```python
from build123d import *

# Parameters (mm, degrees)
SKETCH1_R           = 1
BOSS_EXTRUDE1_DEPTH = 9
SKETCH2_R           = 2
SKETCH2_R_2         = 1
BOSS_EXTRUDE3_DEPTH = 4
SKETCH3_R           = 2
BOSS_EXTRUDE4_DEPTH = 12.3
SKETCH4_W           = 8
SKETCH4_H           = 2.3
CUT_EXTRUDE1_DEPTH  = 100


with BuildPart() as part:
    # Sketch1 → Boss-Extrude1 (new body)
    with BuildSketch(Plane.XY):
        with BuildLine():
            Line((37.44618629, 199.100176708), (21.157913115, 198.645068222))
            ThreePointArc((21.157913115, 198.645068222), (19.402812913, 197.854741355), (18.729526359, 196.051500247))
            Line((18.729526359, 196.051500247), (19.122128495, 185.677380061))
            ThreePointArc((19.122128495, 185.677380061), (19.911642331, 183.946998209), (21.690165088, 183.272898624))
            Line((21.690165088, 183.272898624), (46.213174666, 183.958092791))
            ThreePointArc((46.213174666, 183.958092791), (47.16140114, 184.173792868), (47.955590742, 184.734972736))
            Line((47.955590742, 184.734972736), (53.340647935, 190.401756173))
            Line((53.340647935, 190.401756173), (50.421306908, 190.401756173))
            ThreePointArc((50.421306908, 190.401756173), (49.61024665, 190.536976848), (48.886924084, 190.928011166))
            Line((48.886924084, 190.928011166), (39.050394032, 198.574897009))
            ThreePointArc((39.050394032, 198.574897009), (38.293965035, 198.977028229), (37.44618629, 199.100176708))
        make_face()
        with Locations((20.799047924, 194.252293006)):
            Circle(SKETCH1_R, mode=Mode.SUBTRACT)
        with Locations((38.792906294, 194.755057023)):
            Circle(SKETCH1_R, mode=Mode.SUBTRACT)
        with Locations((39.095459561, 186.760388464)):
            Circle(SKETCH1_R, mode=Mode.SUBTRACT)
        with Locations((21.101601191, 186.257624448)):
            Circle(SKETCH1_R, mode=Mode.SUBTRACT)
    extrude(amount=BOSS_EXTRUDE1_DEPTH)

    # Sketch2 → Boss-Extrude3 (add)
    with BuildSketch(Plane.XY.offset(9)):
        with BuildLine():
            Line((61.820501213, 210.938669532), (45.388864845, 193.647390819))
            Line((45.388864845, 193.647390819), (48.886924084, 190.928011166))
            ThreePointArc((48.886924084, 190.928011166), (49.61024665, 190.536976848), (50.421306908, 190.401756173))
            Line((50.421306908, 190.401756173), (53.340647935, 190.401756173))
            Line((53.340647935, 190.401756173), (67.619672397, 205.427806299))
            ThreePointArc((67.619672397, 205.427806299), (67.475518422, 211.082823507), (61.820501213, 210.938669532))
        make_face()
        with Locations((53.698360337, 196.584895548)):
            Circle(SKETCH2_R, mode=Mode.SUBTRACT)
        with Locations((64.720086805, 208.183237915)):
            Circle(SKETCH2_R, mode=Mode.SUBTRACT)
        with BuildLine():
            Line((37.44618629, 199.100176708), (25.44618629, 198.764886296))
            Line((25.44618629, 198.764886296), (20.867726047, 195.249931876))
            ThreePointArc((20.867726047, 195.249931876), (21.530032918, 194.934686542), (21.799047924, 194.252293006))
            ThreePointArc((21.799047924, 194.252293006), (20.702907489, 193.256925226), (19.817533891, 194.443683189))
            Line((19.817533891, 194.443683189), (18.819373463, 193.677380061))
            Line((18.819373463, 193.677380061), (19.122128495, 185.677380061))
            ThreePointArc((19.122128495, 185.677380061), (19.911642331, 183.946998209), (21.690165088, 183.272898624))
            Line((21.690165088, 183.272898624), (46.213174666, 183.958092791))
            ThreePointArc((46.213174666, 183.958092791), (47.16140114, 184.173792868), (47.955590742, 184.734972736))
            Line((47.955590742, 184.734972736), (53.340647935, 190.401756173))
            Line((53.340647935, 190.401756173), (50.421306908, 190.401756173))
            ThreePointArc((50.421306908, 190.401756173), (49.61024665, 190.536976848), (48.886924084, 190.928011166))
            Line((48.886924084, 190.928011166), (45.388864845, 193.647390819))
            Line((45.388864845, 193.647390819), (39.050394032, 198.574897009))
            ThreePointArc((39.050394032, 198.574897009), (38.293965035, 198.977028229), (37.44618629, 199.100176708))
        make_face()
        with Locations((21.101601191, 186.257624448)):
            Circle(SKETCH2_R_2, mode=Mode.SUBTRACT)
        with Locations((39.095459561, 186.760388464)):
            Circle(SKETCH2_R_2, mode=Mode.SUBTRACT)
        with Locations((38.792906294, 194.755057023)):
            Circle(SKETCH2_R_2, mode=Mode.SUBTRACT)
    extrude(amount=BOSS_EXTRUDE3_DEPTH)

    # Sketch3 → Boss-Extrude4 (add)
    with BuildSketch(Plane.XY.offset(13)):
        with BuildLine():
            Line((67.619672397, 205.427806299), (56.597945929, 193.829463931))
            ThreePointArc((56.597945929, 193.829463931), (50.94292872, 193.685309956), (50.798774745, 199.340327165))
            Line((50.798774745, 199.340327165), (61.820501213, 210.938669532))
            ThreePointArc((61.820501213, 210.938669532), (67.475518422, 211.082823507), (67.619672397, 205.427806299))
        make_face()
        with Locations((64.720086805, 208.183237915)):
            Circle(SKETCH3_R, mode=Mode.SUBTRACT)
        with Locations((53.698360337, 196.584895548)):
            Circle(SKETCH3_R, mode=Mode.SUBTRACT)
    extrude(amount=BOSS_EXTRUDE4_DEPTH)

    # Sketch4 → Cut-Extrude1 (cut)
    with BuildSketch(Plane(origin=(26.111576718, 0.988176406, 0), x_dir=(0, 0, 1), z_dir=(-0.99928467, -0.037817308, 0))):
        with Locations((17.15, 208.436778709)):
            Rectangle(SKETCH4_W, SKETCH4_H)
    extrude(amount=-CUT_EXTRUDE1_DEPTH, mode=Mode.SUBTRACT)


solid = part.part
```
Geometry check sheet. Reference: the model listing, model coordinates, mm. A direction names the side the tool comes from. Coordinates: 2 decimals unless noted, no trailing zeros. Loops run counter-clockwise (first coordinate to the right, second up) from the corner with the lowest first, then second, coordinate; pieces in that order, holes last.
Item 1: Sectioned sample at A-A, the plane z = 11.25. Record the boundary of the cut face in (x, y), then the cut area to 3 significant figures.
Item 2: Thickness scan on line 1 (Z direction, x = 40, y = 187.75); line 2 (Y direction, x = 65, z = 13); line 3 (X direction, y = 195.5, z = 23.75). Record the ranges inside material, lowest first.
Item 3: Sectioned sample at B-B, the plane x = 54. Record the boundary of the cut face in (y, z).
Item 4: Release check for a two-part mould opening along Z. For faces 1 (the face through (38.58, 193.78, 6.41)), 2 (the face through (62.118, 209.786, 17.094)), 3 (the face through (57, 201, 9)) record: released by +Z, released by -Z, zero draft, split by the parting line, or undercut.
Item 5: Sectioned sample at D-D, the plane z = 23.75. Record the boundary of the cut face in (x, y), then the cut area to 3 significant figures.
Item 6: Go/stop test with flat-tipped pins: pin 1 Ø10 at (y, z) = (209, 20) entering from -X; pin 2 Ø2.5 at (x, y) = (63, 210.5) entering from -Z; pin 3 Ø12 at (x, z) = (46.5, 19.5) entering from -Y; pin 4 Ø1.8 at (x, y) = (21.1, 186.26) entering from -Z. Record where each tip stops, or that it passes through.
Item 7: Access from +Z, -Z, +X, -X, +Y, -Y to the whole of each face (thin tool, end or side, straight path). Record for faces 4 (the face through (38.31, 198.97, 6.41)), 5 (the face through (52, 190.402, 4)), 6 (the face through (68.684, 208.721, 17.036)), 7 (the face through (47.15, 184.17, 6.41)), 8 (the face through (19.33, 194.07, 10.97)).
Item 8: Sectioned sample at C-C, the plane z = 20. Record the boundary of the cut face in (x, y), then the cut area to 3 significant figures.
Check result:
1. outline: (18.82, 193.68) - (19.12, 185.68) arc R2.5 ccw to (21.69, 183.27) - (46.21, 183.96) arc R2.5 ccw to (47.96, 184.73) - (67.62, 205.43) arc R4 ccw to (61.82, 210.94) - (45.39, 193.65) - (39.05, 198.57) arc R2.5 ccw to (37.45, 199.1) - (25.45, 198.76) - (20.87, 195.25) arc R1 cw (long way) to (19.82, 194.44) - close; hole circle Ø2 at (21.1, 186.26); hole circle Ø2 at (38.79, 194.76); hole circle Ø2 at (39.1, 186.76); hole circle Ø4 at (53.7, 196.58); hole circle Ø4 at (64.72, 208.18)
1. area: 579 mm2
2. line 1: z = 0 to 13
2. line 2: y = 202.67 to 206.2, 210.16 to 212.17
2. line 3: x = 49.85 to 52.02, 55.38 to 58.19
3. outline: (191.1, 9) - (194.61, 9) - (194.61, 25.3) - (192.6, 25.3) - (192.6, 13) - (191.1, 13) - close; (198.56, 9) - (202.71, 9) - (202.71, 25.3) - (198.56, 25.3) - close
4. face 1: zero draft
4. face 2: undercut
4. face 3: released by -Z
5. outline: (50.8, 199.34) arc R4 ccw to (56.6, 193.83) - (67.62, 205.43) arc R4 ccw to (61.82, 210.94) - close; hole circle Ø4 at (53.7, 196.58); hole circle Ø4 at (64.72, 208.18)
5. area: 153 mm2
6. pin 1: stops at x = 55.23
6. pin 2: stops at z = 9
6. pin 3: stops at y = 192.77
6. pin 4: passes through
7. face 4: +Z, -Z, +Y
7. face 5: -Z, +X, +Y
7. face 6: +Z, -Z
7. face 7: +Z, -Z, +X, -Y
7. face 8: +Z, -X, +Y
8. outline: (50.8, 199.34) arc R4 ccw to (56.6, 193.83) - (67.62, 205.43) arc R4 ccw to (68.27, 210.02) - (65.71, 209.92) arc R2 cw (long way) to (63.6, 209.84) - (60.67, 209.73) - close; hole circle Ø4 at (53.7, 196.58)
8. area: 141 mm2
